Source: CAD feature listing. Evaluate the final solid. Frame: model axes, mm. Face numbers are marked on the shaded views. A direction names the side the tool comes from. Give positions to 0.01 mm unless a question says otherwise; leave off trailing zeros. Loops run counter-clockwise (first coordinate to the right, second up) from the corner with the lowest first, then second, coordinate; pieces in that order, holes last.
from build123d import *

# Parameters (mm, degrees)
F1_ANGLE = 180
F3_DEPTH = 25.4
F4_R     = 1.27
F5_DEPTH = 1.27
F6_R     = 1.27
F7_DEPTH = 1.27


with BuildPart() as f1:
    # F0 (on Front) → F1 (revolve)
    with BuildSketch(Plane.XZ):
        Polygon((0, -19.05), (0, 19.05), (-10.16, 19.05), (-10.16, 11.43), (-6.35, 11.43), (-6.35, 3.81), (-10.16, 3.81), (-10.16, -3.81), (-6.35, -3.81), (-6.35, -11.43), (-10.16, -11.43), (-10.16, -19.05), align=None)
    revolve(axis=Axis((0, 0, 0), (0, 0, 1)), revolution_arc=F1_ANGLE)

    # F2 (on Top) → F3 (cut, symmetric)
    with BuildSketch(Plane.XY):
        with BuildLine():
            ThreePointArc((-5.08, 0), (0, -5.08), (5.08, 0))
            Line((5.08, 0), (-5.08, 0))
        make_face()
    extrude(amount=F3_DEPTH, both=True, mode=Mode.SUBTRACT)

    # F4 (on Front) → F5 (join)
    with BuildSketch(Plane.XZ):
        with Locations((7.62, 15.24)):
            Circle(F4_R)
        with Locations((7.62, -15.24)):
            Circle(F4_R)
    extrude(amount=-F5_DEPTH)

    # F6 (on Front) → F7 (cut)
    with BuildSketch(Plane.XZ):
        with Locations((-7.62, 15.24)):
            Circle(F6_R)
        with Locations((-7.62, -15.24)):
            Circle(F6_R)
    extrude(amount=F7_DEPTH, mode=Mode.SUBTRACT)


solid = f1.part
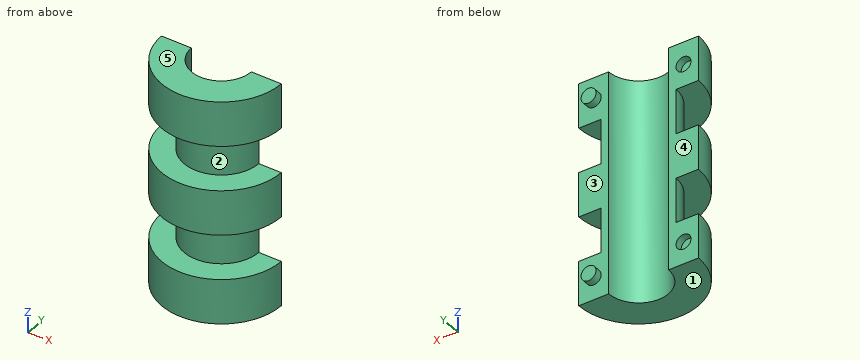
1) Cut plane C-C (z = -15.24). Return loops of the section in (x, y).
Checks:
outline: (-10.16, 0) arc R10.16 ccw to (10.16, 0) - (8.89, 0) - (8.89, 1.27) - (6.35, 1.27) - (6.35, 0) - (5.08, 0) arc R5.08 cw to (-5.08, 0) - (-6.35, 0) - (-6.35, -1.27) - (-8.89, -1.27) - (-8.89, 0) - close
2) Cut plane A-A (y = -7.5). Return loops of the section in (x, z), and give its area (3 significant figures).
Checks:
outline: (-6.85, -19.05) - (6.85, -19.05) - (6.85, -11.43) - (-6.85, -11.43) - close; (-6.85, -3.81) - (6.85, -3.81) - (6.85, 3.81) - (-6.85, 3.81) - close; (-6.85, 11.43) - (6.85, 11.43) - (6.85, 19.05) - (-6.85, 19.05) - close
area: 313 mm2
3) Cut plane D-D (x = -0.75). Return loops of the section in (y, z).
Checks:
outline: (-10.13, -19.05) - (-5.02, -19.05) - (-5.02, 19.05) - (-10.13, 19.05) - (-10.13, 11.43) - (-6.31, 11.43) - (-6.31, 3.81) - (-10.13, 3.81) - (-10.13, -3.81) - (-6.31, -3.81) - (-6.31, -11.43) - (-10.13, -11.43) - close
4) Ray query, probe 1 along Z at (x, y) = (-7.62, -0.45); probe 2 along Z at (x, y) = (-6.5, -2); probe 3 along X at (y, z) = (-0.75, -15). Return the intervals inside material, ascending.
Checks:
probe 1: z = -19.05 to -16.51, -13.97 to -11.43, -3.81 to 3.81, 11.43 to 13.97, 16.51 to 19.05
probe 2: z = -19.05 to -11.43, -3.81 to 3.81, 11.43 to 19.05
probe 3: x = -10.13 to -8.87, -6.37 to -5.02, 5.02 to 10.13
5) Cut plane B-B (x = -7.62). Return loops of the section in (y, z), and give its area (3 significant figures).
Checks:
outline: (-6.72, -19.05) - (0, -19.05) - (0, -16.51) - (-1.27, -16.51) - (-1.27, -13.97) - (0, -13.97) - (0, -11.43) - (-6.72, -11.43) - close; (-6.72, -3.81) - (0, -3.81) - (0, 3.81) - (-6.72, 3.81) - close; (-6.72, 11.43) - (0, 11.43) - (0, 13.97) - (-1.27, 13.97) - (-1.27, 16.51) - (0, 16.51) - (0, 19.05) - (-6.72, 19.05) - close
area: 147 mm2
6) Contact query for flat-ended pins moving along their axis: P1, Ø0.8, axis at x = -8, z = -15, coming from the +Y side; P2, Ø5, axis at y = -4.5, z = 6.5, coming from the -X side; P3, Ø4, axis at x = -7.62, z = -15.24, coming from the -Y side. Output: stop coordinate, or through.
Checks:
P1: stops at y = -1.27
P2: stops at x = -6.03
P3: stops at y = -8.46
7) Reachability of the marked faces 1 and 2 from +Z, -Z, +X, -X, +Y, -Y: full face, straight path, thin tool, end or side. Return the list, or none.
Checks:
face 1: -Z, +X, -X, +Y, -Y
face 2: -Y
8) Pull-direction query (Z, two-part tool) for the marked faces 3, 4 and 5; classes: released by +Z, released by -Z, zero draft, split by the parting line, or undercut.
Checks:
face 3: undercut
face 4: zero draft
face 5: released by +Z
